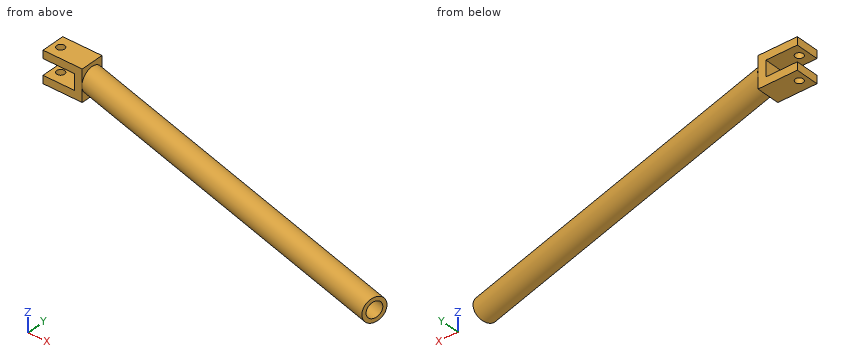
from build123d import *

# Parameters (mm, degrees)
SWEEP1_START         = -25.4
SWEEP1_OUTLINE_R     = 19.05
SWEEP1_DEPTH         = 635
CUT_SWEEP1_START     = -25.4
CUT_SWEEP1_OUTLINE_R = 12.7
CUT_SWEEP1_DEPTH     = 635
SKETCH25_R           = 57.15
CUT_EXTRUDE1_DEPTH   = 620.637672354
SKETCH26_W           = 50.8
SKETCH26_H           = 38.1
BOSS_EXTRUDE1_DEPTH  = 12.7
SKETCH27_W           = 12.7
SKETCH27_H           = 38.1
BOSS_EXTRUDE2_DEPTH  = 50.8
SKETCH28_R           = 6.35
CUT_EXTRUDE2_DEPTH   = 622.424639437


# Read off the part's stored shape, not the designer's step: Sweep1, Cut-Sweep1
with BuildPart() as part:
    # Sweep1 outline → Sweep1 (new body)
    with BuildSketch(Plane(origin=(0, 0, 0), x_dir=(0.2588190451025211, 0.9659258262890682, 0), z_dir=(0.9659258262890682, -0.2588190451025211, 0)).offset(SWEEP1_START)):
        Circle(SWEEP1_OUTLINE_R)
    extrude(amount=SWEEP1_DEPTH)

    # Cut-Sweep1 outline → Cut-Sweep1 (cut)
    with BuildSketch(Plane(origin=(0, 0, 0), x_dir=(0.2588190451025211, 0.9659258262890682, 0), z_dir=(0.9659258262890682, -0.2588190451025211, 0)).offset(CUT_SWEEP1_START)):
        Circle(CUT_SWEEP1_OUTLINE_R)
    extrude(amount=CUT_SWEEP1_DEPTH, mode=Mode.SUBTRACT)

    # Sketch25 → Cut-Extrude1 (cut, through all)
    with BuildSketch(Plane(origin=(0, 0, 0), x_dir=(0, 0, -1), z_dir=(1, 0, 0))):
        Circle(SKETCH25_R)
    extrude(amount=-CUT_EXTRUDE1_DEPTH, mode=Mode.SUBTRACT)

    # Sketch26 → Boss-Extrude1 (add)
    with BuildSketch(Plane(origin=(0, 0, 0), x_dir=(0, 0, -1), z_dir=(1, 0, 0))):
        Rectangle(SKETCH26_W, SKETCH26_H)
    extrude(amount=-BOSS_EXTRUDE1_DEPTH)

    # Sketch27 → Boss-Extrude2 (add)
    with BuildSketch(Plane.ZY.offset(12.7)):
        with Locations((19.05, 0)):
            Rectangle(SKETCH27_W, SKETCH27_H)
        with Locations((-19.05, 0)):
            Rectangle(SKETCH27_W, SKETCH27_H)
    extrude(amount=BOSS_EXTRUDE2_DEPTH)

    # Sketch28 → Cut-Extrude2 (cut, through all)
    with BuildSketch(Plane.XY.offset(25.4)):
        with Locations((-50.8, 0)):
            Circle(SKETCH28_R)
    extrude(amount=-CUT_EXTRUDE2_DEPTH, mode=Mode.SUBTRACT)


solid = part.part
Part model, mm, in its own coordinate system. Give positions to 0.01 mm unless a question says otherwise; leave off trailing zeros. Loops run counter-clockwise (first coordinate to the right, second up) from the corner with the lowest first, then second, coordinate; pieces in that order, holes last.
(1) Band-saw the part on B-B (y = 0). Count the separate pieces of the cut face and the enclosed holes in it, and give its area (3 significant figures).
Return value:
separate pieces: 3
enclosed holes: 1
area: 2,840 mm2
(2) Drill centre lines: line 1 along Y through (x, z) = (-50.8, 21); line 2 along Z through (x, y) = (206, -53); line 3 along Z through (x, y) = (260.5, -78). Where is each one in solid material? Low to high.
Return value:
line 1: y = -19.05 to -6.35, 6.35 to 19.05
line 2: z = -18.93 to -12.52, 12.52 to 18.93
line 3: z = -17.33 to -9.93, 9.93 to 17.33
(3) Pin check, flat tips, straight feed: pin 1 (3 mm diameter, centred on x = 43.5, z = -17.5, fed in from +Y); pin 2 (2 mm diameter, centred on x = 286.5, z = -17, fed in from +Y); pin 3 (7.5 mm diameter, centred on y = -7, z = 2.5, fed in from -X). Stop position of each tip, or through.
Return value:
pin 1: stops at y = -0.92
pin 2: stops at y = -66.04
pin 3: stops at x = -12.7
(4) Band-saw the part on A-A (x = -50.8). Write the cut outline in (y, z), and give its area (3 significant figures).
Return value:
outline: (-19.05, -25.4) - (-6.35, -25.4) - (-6.35, -12.7) - (-19.05, -12.7) - close; (-19.05, 12.7) - (-6.35, 12.7) - (-6.35, 25.4) - (-19.05, 25.4) - close; (6.35, -25.4) - (19.05, -25.4) - (19.05, -12.7) - (6.35, -12.7) - close; (6.35, 12.7) - (19.05, 12.7) - (19.05, 25.4) - (6.35, 25.4) - close
area: 645 mm2
